CAD build for the part. Positions are in the model's coordinates, mm. A direction names the side the tool comes from. Give positions to 0.01 mm unless a question says otherwise; leave off trailing zeros. Write each loop counter-clockwise with the first axis right and the second up, starting at its lowest first coordinate (ties: lowest second). Pieces come first, ordered by that corner, then holes. Notation, with made-up numbers: M 28.25,78 L 35.25,78 A17 cw 35.25,93 Z; hole C 11.25,44 d2. An arc over 180 degrees is marked long. One line per question, with ' | ' between items. Start each with the question number.
1. Cut at A-A, the plane y = -5.75. Write the cut outline in (x, z), then the cut area to 3 significant figures.
2. Cut at C-C, the plane z = 8. Write the cut outline in (x, y), then the cut area to 3 significant figures.
3. Which spindle directions (+Z, -Z, +X, -X, +Y, -Y) get a long thin tool onto all of the face, cutting with end or side? Do faces 1 (the face through (9.5, 0, 10)), 2 (the face through (2, 5, 23)), 3 (the face through (0, 6.5, 10)). Say none if no direction does.
4. Cut at B-B, the plane x = -4. Write the cut outline in (y, z).
5. Wall check: L1, parallel to Z at x = 7.5, y = -6; L2, parallel to X at y = 4.5, z = 3.5; L3, parallel to Y at x = -3, z = 1.5. Give the ranges that are in metal, low to high.
6. Cut at D-D, the plane y = 4.5. Write the cut outline in (x, z).
7. Flat gauge pins, fed straight in: pin 1 (1.5 mm diameter, centred on x = 4, z = 10.5, fed in from -Y); pin 2 (4 mm diameter, centred on y = 2, z = 9.5, fed in from +X); pin 3 (5 mm diameter, centred on y = -2, z = 14, fed in from -X). Where does each tip first touch, or does it go through?
```python
from build123d import *

# Parameters (mm, degrees)
SKETCH1_W                = 19
SKETCH1_H                = 13
BOSS_EXTRUDE1_DEPTH      = 20
SKETCH2_W                = 21
SKETCH2_H                = 15
BOSS_EXTRUDE2_DEPTH      = 2
BOSS_EXTRUDE3_DEPTH      = 5
BOSS_EXTRUDE3_DEPTH_BACK = 5


with BuildPart() as part:
    # Sketch1 → Boss-Extrude1 (new body)
    with BuildSketch(Plane.XY):
        Rectangle(SKETCH1_W, SKETCH1_H)
    extrude(amount=BOSS_EXTRUDE1_DEPTH)

    # Sketch2 → Boss-Extrude2 (add)
    with BuildSketch(Plane.XY.offset(20)):
        Rectangle(SKETCH2_W, SKETCH2_H)
    extrude(amount=BOSS_EXTRUDE2_DEPTH)

    # Sketch3 → Boss-Extrude3 (add, two sides)
    with BuildSketch(Plane(origin=(0, 0, 0), x_dir=(1, 0, 0), z_dir=(0, 1, 0))) as boss_extrude3_sk:
        Polygon((-7.218671047, -22), (-7.218671047, -22.66914067), (6.952686856, -24.857910608), (7.694642767, -22), align=None)
    extrude(amount=BOSS_EXTRUDE3_DEPTH)
    extrude(boss_extrude3_sk.sketch, amount=-BOSS_EXTRUDE3_DEPTH_BACK)


solid = part.part
```
Here are the results:
1) outline: M -10.5,20 L -9.5,20 L -9.5,0 L 9.5,0 L 9.5,20 L 10.5,20 L 10.5,22 L -10.5,22 Z | area: 422 mm^2
2) outline: M -9.5,-6.5 L 9.5,-6.5 L 9.5,6.5 L -9.5,6.5 Z | area: 247 mm^2
3) face 1: -Z, +X, +Y, -Y | face 2: +Z, +X, -X, +Y | face 3: -Z, +X, -X, +Y
4) outline: M -7.5,20 L -6.5,20 L -6.5,0 L 6.5,0 L 6.5,20 L 7.5,20 L 7.5,22 L 5,22 L 5,23.17 L -5,23.17 L -5,22 L -7.5,22 Z
5) L1: 0 to 22 | L2: -9.5 to 9.5 | L3: -6.5 to 6.5
6) outline: M -10.5,20 L -9.5,20 L -9.5,0 L 9.5,0 L 9.5,20 L 10.5,20 L 10.5,22 L 7.69,22 L 6.95,24.86 L -7.22,22.67 L -7.22,22 L -10.5,22 Z
7) pin 1: y = -6.5 | pin 2: x = 9.5 | pin 3: x = -9.5
